```python
from build123d import *

# Parameters (mm, degrees)
F0_R     = 3
F1_DEPTH = 25
F4_W     = 40
F4_H     = 30
F5_DEPTH = 5
F7_R     = 2


with BuildPart() as f1:
    # F0 (on Top) → F1 (new body)
    with BuildSketch(Plane.XY):
        with Locations((-12, 9)):
            Circle(F0_R)
    extrude(amount=F1_DEPTH)


with BuildPart() as f2_1:
    # F2: instance of F1
    add(f1.part.mirror(Plane.YZ))


with BuildPart() as f3_1:
    # F3: instance of F1
    add(f1.part.mirror(Plane.XZ))


with BuildPart() as f3_2:
    # F3: instance of F2_1
    add(f2_1.part.mirror(Plane.XZ))


with BuildPart() as f5:
    # F4 (on Top) → F5 (new body)
    with BuildSketch(Plane.XY):
        Rectangle(F4_W, F4_H)
    extrude(amount=F5_DEPTH)

    # F6: cut F1, F2_1, F3_1, F3_2
    add(f1.part, mode=Mode.SUBTRACT)
    add(f2_1.part, mode=Mode.SUBTRACT)
    add(f3_1.part, mode=Mode.SUBTRACT)
    add(f3_2.part, mode=Mode.SUBTRACT)

    # F7
    f7_edges = [f5.edges().sort_by_distance(p)[0] for p in [
        (0, -15, 5),
        (-20, 0, 5),
        (0, 15, 5),
        (20, 0, 5),
    ]]
    fillet(f7_edges, radius=F7_R)


solid = f5.part
```
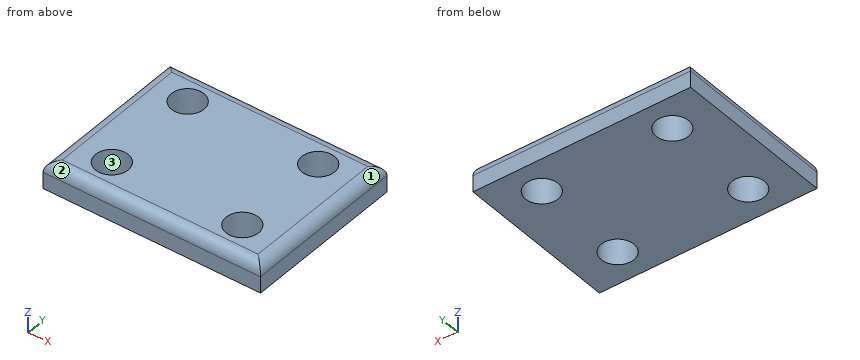
Verification items for the finished model (mm, model axes). Face numbers are marked on the shaded views. Round coordinates to 2 decimals unless told otherwise and drop trailing zeros. Order: outer loops, then holes, each group sorted by start corner. A loop starts at its lowest first (then second) coordinate and runs counter-clockwise, first axis right, second up. Notation, with made-up numbers: (34.5, -5) -> (40.5, -5) arc R33 cw to (40.5, 29) -> close; hole circle Ø8 at (83.25, 63.5). An arc over 180 degrees is marked (long way). Put each result on its own line as item: value. Start each with the question number.
(1) Section check B-B (y = 9). Enter the section's corners in (x, z), then the cut area to 3 significant figures.
(2) Draft check along X on the marked faces 1, 2 and 3. Enter one of: +X half, -X half, draft (parallel to the pull), parting line (faces both ways), or undercut.
(3) Material ranges on line 1 along Y through (x, z) = (12, 2.1); line 2 along X through (y, z) = (-9, 1.75); line 3 along Y through (x, z) = (-10, 2), recorded low to high.
(4) Depth check by flat-ended pin: pin 1 Ø8 at (x, y) = (12, -9) entering from +Z. Enter the tip coordinate at first touch or a pass-through.
(5) Section check C-C (z = 2). Enter the section's corners in (x, y), then the cut area to 3 significant figures.
(6) Section check A-A (x = -12). Enter the section's corners in (y, z), then the cut area to 3 significant figures.
Completed:
1. outline: (-20, 0) -> (-15, 0) -> (-15, 5) -> (-18, 5) arc R2 ccw to (-20, 3) -> close; (-9, 0) -> (9, 0) -> (9, 5) -> (-9, 5) -> close; (15, 0) -> (20, 0) -> (20, 3) arc R2 ccw to (18, 5) -> (15, 5) -> close
1. area: 138 mm2
2. face 1: +X half
2. face 2: draft
2. face 3: undercut
3. line 1: y = -15 to -12, -6 to 6, 12 to 15
3. line 2: x = -20 to -15, -9 to 9, 15 to 20
3. line 3: y = -15 to -11.24, -6.76 to 6.76, 11.24 to 15
4. pin 1: stops at z = 5
5. outline: (-20, -15) -> (20, -15) -> (20, 15) -> (-20, 15) -> close; hole circle Ø6 at (-12, -9); hole circle Ø6 at (-12, 9); hole circle Ø6 at (12, -9); hole circle Ø6 at (12, 9)
5. area: 1,090 mm2
6. outline: (-15, 0) -> (-12, 0) -> (-12, 5) -> (-13, 5) arc R2 ccw to (-15, 3) -> close; (-6, 0) -> (6, 0) -> (6, 5) -> (-6, 5) -> close; (12, 0) -> (15, 0) -> (15, 3) arc R2 ccw to (13, 5) -> (12, 5) -> close
6. area: 88.3 mm2
